```python
from build123d import *

# Parameters (mm, degrees)
SKETCH1_W               = 276.86
SKETCH1_H               = 154.0256
SKETCH1_W_2             = 260.9596
SKETCH1_H_2             = 138.1252
BOSS_EXTRUDE1_DEPTH     = 9.525
SKETCH2_R               = 3.3655
SKETCH2_R_2             = 3.429
CUT_EXTRUDE1_DEPTH      = 288.52940126
SKETCH3_R               = 1.5875
BOSS_EXTRUDE2_DEPTH     = 3.175
MIRROR2_COPY_1_SKETCH_R = 1.5875
MIRROR2_COPY_1_DEPTH    = 3.175
FILLET1_R               = 1.524
SKETCH4_W               = 25.781
SKETCH4_H               = 13.462
CUT_EXTRUDE2_DEPTH      = 3.175
CUT_EXTRUDE3_REACH      = 214.311
SKETCH5_R               = 1.27


with BuildPart() as part:
    # Sketch1 → Boss-Extrude1 (new body)
    with BuildSketch(Plane.XY):
        Rectangle(SKETCH1_W, SKETCH1_H)
        Rectangle(SKETCH1_W_2, SKETCH1_H_2, mode=Mode.SUBTRACT)
    extrude(amount=BOSS_EXTRUDE1_DEPTH)

    # Sketch2 → Cut-Extrude1 (cut, through all)
    with BuildSketch(Plane(origin=(138.43, 0, 0), x_dir=(0, 0, -1), z_dir=(1, 0, 0))):
        Circle(SKETCH2_R)
        with Locations((0, 34.5313)):
            Circle(SKETCH2_R)
        with Locations((0, -34.5313)):
            Circle(SKETCH2_R_2)
    extrude(amount=-CUT_EXTRUDE1_DEPTH, mode=Mode.SUBTRACT)

    # Sketch3 → Boss-Extrude2 (add)
    with BuildSketch(Plane(origin=(0, 0, 0), x_dir=(-1, 0, 0), z_dir=(0, 0, -1))):
        with BuildLine():
            Line((-138.43, 77.0128), (-138.43, 82.0928))
            ThreePointArc((-138.43, 82.0928), (-133.6675, 86.8553), (-128.905, 82.0928))
            Line((-128.905, 82.0928), (-128.905, 77.0128))
            Line((-128.905, 77.0128), (-138.43, 77.0128))
        make_face()
        with Locations((-133.6675, 82.0928)):
            Circle(SKETCH3_R, mode=Mode.SUBTRACT)
    boss_extrude2 = extrude(amount=-BOSS_EXTRUDE2_DEPTH)

    # Mirror1: Boss-Extrude2 across plane
    add(boss_extrude2.mirror(Plane(origin=(0, 0, 0), x_dir=(0, 0, 1), z_dir=(1, 0, 0))))

    # Mirror2: Boss-Extrude2 across plane
    add(boss_extrude2.mirror(Plane.ZX))

    # Mirror2 copy 1 sketch → Mirror2 copy 1 (add)
    with BuildSketch(Plane(origin=(0, 0, 0), x_dir=(1, 0, 0), z_dir=(0, 0, -1))):
        with BuildLine():
            Line((-138.43, 77.0128), (-138.43, 82.0928))
            ThreePointArc((-138.43, 82.0928), (-133.6675, 86.8553), (-128.905, 82.0928))
            Line((-128.905, 82.0928), (-128.905, 77.0128))
            Line((-128.905, 77.0128), (-138.43, 77.0128))
        make_face()
        with Locations((-133.6675, 82.0928)):
            Circle(MIRROR2_COPY_1_SKETCH_R, mode=Mode.SUBTRACT)
    extrude(amount=-MIRROR2_COPY_1_DEPTH)

    # Fillet1
    fillet1_edges = [part.edges().sort_by_distance(p)[0] for p in [
        (133.6675, -77.0128, 3.175),
        (128.905, -77.0128, 1.5875),
        (-133.6675, -77.0128, 3.175),
        (-128.905, -77.0128, 1.5875),
        (133.6675, 77.0128, 3.175),
        (128.905, 77.0128, 1.5875),
        (-133.6675, 77.0128, 3.175),
        (-128.905, 77.0128, 1.5875),
    ]]
    fillet(fillet1_edges, radius=FILLET1_R)

    # Sketch4 → Cut-Extrude2 (cut)
    with BuildSketch(Plane(origin=(0, 77.0128, 0), x_dir=(1, 0, 0), z_dir=(0, 1, 0))):
        Rectangle(SKETCH4_W, SKETCH4_H)
    cut_extrude2 = extrude(amount=-CUT_EXTRUDE2_DEPTH, mode=Mode.SUBTRACT)

    # Sketch5 → Cut-Extrude3 (cut, up to next)
    with BuildSketch(Plane(origin=(0, 73.8378, 0), x_dir=(1, 0, 0), z_dir=(0, 1, 0)), mode=Mode.PRIVATE) as cut_extrude3_sk1:
        with Locations(Location((6.35, -3.175, 0), (0, 0, 270))):
            Circle(SKETCH5_R)
    cut_extrude3_tool1 = extrude(cut_extrude3_sk1.sketch, amount=-CUT_EXTRUDE3_REACH, mode=Mode.PRIVATE) & part.part
    # Sketch5 → Cut-Extrude3 (cut, up to next)
    with BuildSketch(Plane(origin=(0, 73.8378, 0), x_dir=(1, 0, 0), z_dir=(0, 1, 0)), mode=Mode.PRIVATE) as cut_extrude3_sk2:
        with Locations(Location((-6.35, -3.175, 0), (0, 0, 270))):
            Circle(SKETCH5_R)
    cut_extrude3_tool2 = extrude(cut_extrude3_sk2.sketch, amount=-CUT_EXTRUDE3_REACH, mode=Mode.PRIVATE) & part.part
    cut_extrude3_1 = cut_extrude3_tool1.solids().sort_by_distance((6.35, 73.8378, 3.175))[0]
    add(cut_extrude3_1, mode=Mode.SUBTRACT)
    cut_extrude3_2 = cut_extrude3_tool2.solids().sort_by_distance((-6.35, 73.8378, 3.175))[0]
    add(cut_extrude3_2, mode=Mode.SUBTRACT)
    cut_extrude3 = cut_extrude3_1 + cut_extrude3_2  # Cut-Extrude3 as one shape, for the pattern or mirror that repeats it

    # Mirror3: Cut-Extrude2, Cut-Extrude3 across plane
    add(cut_extrude2.mirror(Plane.ZX), mode=Mode.SUBTRACT)
    add(cut_extrude3.mirror(Plane.ZX), mode=Mode.SUBTRACT)


solid = part.part
```
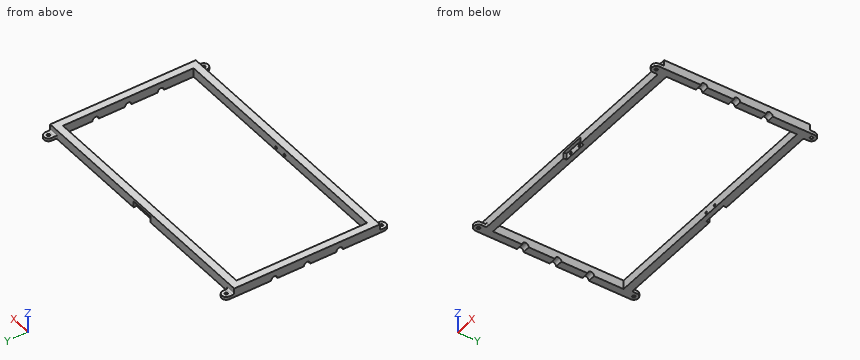
The model under review builds one solid part; all positions refer to its coordinate system, in mm. Round coordinates to 2 decimals unless told otherwise and drop trailing zeros. Write each loop counter-clockwise with the first axis right and the second up, starting at its lowest first coordinate (ties: lowest second). Pieces come first, ordered by that corner, then holes. Notation, with made-up numbers: M -29.75,7.5 L -16.75,7.5 A10 cw -16.75,24.5 Z; hole C -14.75,27 d10. An arc over 180 degrees is marked long. Use CSV: the item, a comma, the result in double quotes. Start each with the question number.
(1) For line 1 along Y through (x, z) = (-76.5, 3.5); line 2 along X through (y, z) = (-65.5, 5.25); line 3 along X through (y, z) = (-78.5, 2.75), list the stretches that pass through material, from the lowest coordinate up.
(2) Clearance check with flat-ended pins moving along their axes: P1, Ø3, axis at x = 6.35, z = 3.175, coming from the -Y side; P2, Ø6.5, axis at x = -136, y = 81.5, coming from the +Z side; P3, Ø3, axis at x = 45.5, z = 6.5, coming from the +Y side. State where each tip first meets the part, or that it passes through.
(3) We need section A-A, the plane y = -42. State the section outline as (x, z) points (3 decimals).
(4) We need section B-B, the plane x = -112. State the section outline as (y, z) points (3 decimals).
Findings:
1,line 1,"-77.01 to -69.06, 69.06 to 77.01"
1,line 2,"-138.43 to -130.48, 130.48 to 138.43"
1,line 3,"-138.43 to -128.9, 128.9 to 138.43"
2,P1,"y = -73.84"
2,P2,"z = 3.2"
2,P3,"y = 77.01"
3,outline,"M -138.43,0 L -130.48,0 L -130.48,9.525 L -138.43,9.525 Z; M 130.48,0 L 138.43,0 L 138.43,9.525 L 130.48,9.525 Z"
4,outline,"M -77.013,0 L -69.063,0 L -69.063,9.525 L -77.013,9.525 Z; M 69.063,0 L 77.013,0 L 77.013,9.525 L 69.063,9.525 Z"
